For this review, take the finished solid that the model builds, in its own axes (mm). Face numbers are marked on the shaded views. Round coordinates to 2 decimals unless told otherwise and drop trailing zeros. Write each loop counter-clockwise with the first axis right and the second up, starting at its lowest first coordinate (ties: lowest second). Pieces come first, ordered by that corner, then holes.
from build123d import *

# Parameters (mm, degrees)
SKETCH_W        = 90
SKETCH_H        = 60
SKETCH_W_2      = 68
SKETCH_H_2      = 52
PAD_DEPTH       = 1
SKETCH001_W     = 90
SKETCH001_H     = 60
SKETCH001_W_2   = 85
SKETCH001_H_2   = 55.4
PAD001_DEPTH    = 1
SKETCH002_W     = 87.5
SKETCH002_H     = 57
SKETCH002_W_2   = 85
SKETCH002_H_2   = 55.4
PAD002_DEPTH    = 2
SKETCH003_W     = 5
SKETCH003_H     = 1
POCKET_DEPTH    = 58.501
POCKET001_DEPTH = 4.001
CHAMFER_SIZE    = 0.4


with BuildPart() as part:
    # Sketch → Pad (new body)
    with BuildSketch(Plane.XY):
        Rectangle(SKETCH_W, SKETCH_H)
        Rectangle(SKETCH_W_2, SKETCH_H_2, mode=Mode.SUBTRACT)
    extrude(amount=PAD_DEPTH)

    # Sketch001 → Pad001 (new body)
    with BuildSketch(Plane.XY.offset(1)):
        Rectangle(SKETCH001_W, SKETCH001_H)
        Rectangle(SKETCH001_W_2, SKETCH001_H_2, mode=Mode.SUBTRACT)
    extrude(amount=PAD001_DEPTH)

    # Sketch002 → Pad002 (new body)
    with BuildSketch(Plane.XY.offset(2)):
        Rectangle(SKETCH002_W, SKETCH002_H)
        Rectangle(SKETCH002_W_2, SKETCH002_H_2, mode=Mode.SUBTRACT)
    extrude(amount=PAD002_DEPTH)

    # Sketch003 → Pocket (cut, through all)
    with BuildSketch(Plane.XZ.offset(28.5)):
        with Locations((-30, 2.5)):
            Rectangle(SKETCH003_W, SKETCH003_H)
        with Locations((0, 2.5)):
            Rectangle(SKETCH003_W, SKETCH003_H)
        with Locations((30, 2.5)):
            Rectangle(SKETCH003_W, SKETCH003_H)
    extrude(amount=-POCKET_DEPTH, mode=Mode.SUBTRACT)

    # Sketch004 → Pocket001 (cut, through all)
    with BuildSketch(Plane(origin=(0, 0, 0), x_dir=(1, 0, 0), z_dir=(0, 0, -1))):
        with BuildLine():
            ThreePointArc((-37.5, 14), (-39.5, 16), (-41.5, 14))
            Line((-41.5, 14), (-41.5, 10))
            ThreePointArc((-41.5, 10), (-39.5, 8), (-37.5, 10))
            Line((-37.5, 14), (-37.5, 10))
        make_face()
        with BuildLine():
            ThreePointArc((-37.5, 0.5), (-39.5, 2.5), (-41.5, 0.5))
            Line((-41.5, 0.5), (-41.5, -3.5))
            ThreePointArc((-41.5, -3.5), (-39.5, -5.5), (-37.5, -3.5))
            Line((-37.5, 0.5), (-37.5, -3.5))
        make_face()
        with BuildLine():
            ThreePointArc((-37.5, -13), (-39.5, -11), (-41.5, -13))
            Line((-41.5, -13), (-41.5, -17))
            ThreePointArc((-41.5, -17), (-39.5, -19), (-37.5, -17))
            Line((-37.5, -13), (-37.5, -17))
        make_face()
    extrude(amount=-POCKET001_DEPTH, mode=Mode.SUBTRACT)

    # Chamfer
    chamfer_edges = [part.edges().sort_by_distance(p)[0] for p in [
        (0, 28.5, 4),
        (0, -28.5, 4),
    ]]
    chamfer(chamfer_edges, length=CHAMFER_SIZE)


solid = part.part
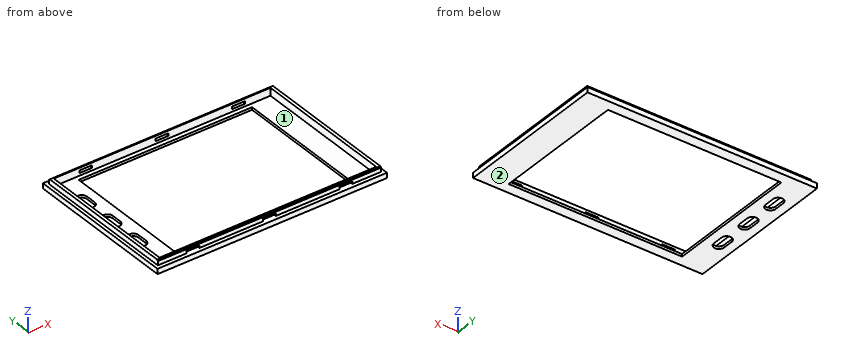
(1) We need section B-B, the plane x = -39.5. Give the boundary of the cut face in (y, z), and give its area (3 significant figures).
Geometry check:
outline: (-30, 0) - (-16, 0) - (-16, 1) - (-27.7, 1) - (-27.7, 4) - (-28.1, 4) - (-28.5, 3.6) - (-28.5, 2) - (-30, 2) - close; (-8, 0) - (-2.5, 0) - (-2.5, 1) - (-8, 1) - close; (5.5, 0) - (11, 0) - (11, 1) - (5.5, 1) - close; (19, 0) - (30, 0) - (30, 2) - (28.5, 2) - (28.5, 3.6) - (28.1, 4) - (27.7, 4) - (27.7, 1) - (19, 1) - close
area: 43.6 mm2
(2) For pin 1 Ø0.6 at (y, z) = (-28, 2.5) entering from -X, flat-tipped, find the tip position at first contact; note if it passes through.
Geometry check:
pin 1: stops at x = -43.75
(3) We need section D-D, the plane x = 1. Give the boundary of the cut face in (y, z), and give its area (3 significant figures).
Geometry check:
outline: (-30, 0) - (-26, 0) - (-26, 1) - (-27.7, 1) - (-27.7, 2) - (-30, 2) - close; (-28.5, 3) - (-27.7, 3) - (-27.7, 4) - (-28.1, 4) - (-28.5, 3.6) - close; (26, 0) - (30, 0) - (30, 2) - (27.7, 2) - (27.7, 1) - (26, 1) - close; (27.7, 3) - (28.5, 3) - (28.5, 3.6) - (28.1, 4) - (27.7, 4) - close
area: 14.0 mm2
(4) We need section C-C, the plane y = -7. Give the boundary of the cut face in (x, z).
Geometry check:
outline: (-45, 0) - (-34, 0) - (-34, 1) - (-42.5, 1) - (-42.5, 4) - (-43.75, 4) - (-43.75, 2) - (-45, 2) - close; (34, 0) - (45, 0) - (45, 2) - (43.75, 2) - (43.75, 4) - (42.5, 4) - (42.5, 1) - (34, 1) - close
(5) For line 1 along X through (y, z) = (-12.5, 0.4); line 2 along Y through (x, z) = (8, 0.6); line 3 along Y through (x, z) = (-17, 3.3), list the stretches that pass through material, from the lowest coordinate up.
Geometry check:
line 1: x = -45 to -41.5, -37.5 to -34, 34 to 45
line 2: y = -30 to -26, 26 to 30
line 3: y = -28.5 to -27.7, 27.7 to 28.5
(6) We need section A-A, the plane y = 15. Give the boundary of the cut face in (x, z).
Geometry check:
outline: (-45, 0) - (-41.5, 0) - (-41.5, 1) - (-42.5, 1) - (-42.5, 4) - (-43.75, 4) - (-43.75, 2) - (-45, 2) - close; (-37.5, 0) - (-34, 0) - (-34, 1) - (-37.5, 1) - close; (34, 0) - (45, 0) - (45, 2) - (43.75, 2) - (43.75, 4) - (42.5, 4) - (42.5, 1) - (34, 1) - close
(7) Mouldability with a two-part tool opening along X and no side actions: class the marked faces 1 and 2 as pulls with the +X half, pulls with the -X half, needs draft (parallel to the pull), parting line crosses it, or undercut.
Geometry check:
face 1: undercut
face 2: needs draft
